```python
from build123d import *

# Parameters (mm, degrees)
BOSS_EXTRUDE1_DEPTH = 40
CUT_EXTRUDE1_REACH  = 4
SKETCH2_R           = 17.5
CUT_EXTRUDE2_REACH  = 4
CUT_EXTRUDE3_REACH  = 4
SKETCH6_R           = 2


with BuildPart() as part:
    # Sketch1 → Boss-Extrude1 (new body)
    with BuildSketch(Plane.XY):
        Polygon((0, 0), (0, 62), (2, 62), (2, 2), (22, 2), (22, 0), align=None)
    extrude(amount=BOSS_EXTRUDE1_DEPTH)

    # Sketch2 → Cut-Extrude1 (cut, up to next)
    with BuildSketch(Plane(origin=(2, 0, 0), x_dir=(0, 0, -1), z_dir=(1, 0, 0)), mode=Mode.PRIVATE) as cut_extrude1_sk1:
        with Locations((-20, 42)):
            Circle(SKETCH2_R)
    cut_extrude1_tool1 = extrude(cut_extrude1_sk1.sketch, amount=-CUT_EXTRUDE1_REACH, mode=Mode.PRIVATE) & part.part
    add(cut_extrude1_tool1.solids().sort_by_distance((2, 42, 20))[0], mode=Mode.SUBTRACT)

    # Sketch5 → Cut-Extrude2 (cut, up to next)
    with BuildSketch(Plane(origin=(2, 0, 0), x_dir=(0, 0, -1), z_dir=(1, 0, 0)), mode=Mode.PRIVATE) as cut_extrude2_sk1:
        with BuildLine():
            Line((-40, 62), (-40, 42))
            ThreePointArc((-40, 42), (-34.142135624, 56.142135624), (-20, 62))
            Line((-20, 62), (-40, 62))
        make_face()
    cut_extrude2_tool1 = extrude(cut_extrude2_sk1.sketch, amount=-CUT_EXTRUDE2_REACH, mode=Mode.PRIVATE) & part.part
    add(cut_extrude2_tool1.solids().sort_by_distance((2, 57.532641, 35.532641))[0], mode=Mode.SUBTRACT)
    # Sketch5 → Cut-Extrude2 (cut, up to next)
    with BuildSketch(Plane(origin=(2, 0, 0), x_dir=(0, 0, -1), z_dir=(1, 0, 0)), mode=Mode.PRIVATE) as cut_extrude2_sk2:
        with BuildLine():
            Line((0, 62), (-20, 62))
            ThreePointArc((-20, 62), (-5.857864376, 56.142135624), (0, 42))
            Line((0, 42), (0, 62))
        make_face()
    cut_extrude2_tool2 = extrude(cut_extrude2_sk2.sketch, amount=-CUT_EXTRUDE2_REACH, mode=Mode.PRIVATE) & part.part
    add(cut_extrude2_tool2.solids().sort_by_distance((2, 57.532641, 4.467359))[0], mode=Mode.SUBTRACT)

    # Sketch6 → Cut-Extrude3 (cut, up to next)
    with BuildSketch(Plane(origin=(0, 2, 0), x_dir=(1, 0, 0), z_dir=(0, 1, 0)), mode=Mode.PRIVATE) as cut_extrude3_sk1:
        with Locations((12, -9)):
            Circle(SKETCH6_R)
    cut_extrude3_tool1 = extrude(cut_extrude3_sk1.sketch, amount=-CUT_EXTRUDE3_REACH, mode=Mode.PRIVATE) & part.part
    add(cut_extrude3_tool1.solids().sort_by_distance((12, 2, 9))[0], mode=Mode.SUBTRACT)
    # Sketch6 → Cut-Extrude3 (cut, up to next)
    with BuildSketch(Plane(origin=(0, 2, 0), x_dir=(1, 0, 0), z_dir=(0, 1, 0)), mode=Mode.PRIVATE) as cut_extrude3_sk2:
        with Locations((12, -31)):
            Circle(SKETCH6_R)
    cut_extrude3_tool2 = extrude(cut_extrude3_sk2.sketch, amount=-CUT_EXTRUDE3_REACH, mode=Mode.PRIVATE) & part.part
    add(cut_extrude3_tool2.solids().sort_by_distance((12, 2, 31))[0], mode=Mode.SUBTRACT)


solid = part.part
```
Read the model definition and answer for the solid it produces. Units are mm, in the model's axes. A direction names the side the tool comes from. Coordinates: 2 decimals unless noted, no trailing zeros. Write each loop counter-clockwise with the first axis right and the second up, starting at its lowest first coordinate (ties: lowest second). Pieces come first, ordered by that corner, then holes. Notation, with made-up numbers: (83.25, 71) - (97.25, 71) arc R17 cw to (97.25, 87) - close; hole circle Ø8 at (38.5, -22). An arc over 180 degrees is marked (long way). Answer as a JSON object with one key per item and string values. Group by question number.
1. A cutting plane is placed at A-A (x = 12). Determine the outline of the cut face in (y, z).
2. The mould has two halves that part along Z. Classify faces 3 (the flat face through (22, 1, 20)), 4 (the cylindrical face through (12, 1, 33)), 5 (the flat face through (1, 15, 0)): +Z half, -Z half, draft (parallel to the pull), parting line (faces both ways), or undercut.
3. Which of the six approach directions +Z, -Z, +X, -X, +Y, -Y give full straight-line access (tool end or side, diameter ignored) to faces 1 (the flat face through (12, 2, 20)), 2 (the cylindrical face through (1.014, 53.827, 32.898))?
4. Consider L1, parallel to Z at x = 12, y = 1.55; L2, parallel to X at y = 1, z = 31; L3, parallel to Y at x = 1.35, z = 20. Determine where each line is inside the solid, lowest interval first. Write a range as [from, to].
5. A cutting plane is placed at D-D (x = 16.25). Determine the outline of the cut face in (y, z).
6. A cutting plane is placed at B-B (z = 5.5). Determine the outline of the cut face in (x, y), plus the area to 3 significant figures.
7. Each of these flat-tipped pins is pushed along its axis until it touches: P1, Ø2, axis at x = 10.5, z = 19.5, coming from the -Y side; P2, Ø3, axis at x = 2.5, z = 33.5, coming from the +Y side; P3, Ø5, axis at x = 10, z = 29.5, coming from the +Y side. Where does it stop, or does it pass through?
8. A cutting plane is placed at C-C (y = 48). Determine the outline of the cut face in (x, z).
Worked out:
{
 "1": {"outline": "(0, 0) - (2, 0) - (2, 7) - (0, 7) - close; (0, 11) - (2, 11) - (2, 29) - (0, 29) - close; (0, 33) - (2, 33) - (2, 40) - (0, 40) - close"},
 "2": {"face 3": "draft", "face 4": "undercut", "face 5": "-Z half"},
 "3": {"face 1": "+Z, -Z, +X, +Y", "face 2": "+X, -X"},
 "4": {"L1": "z = [0, 7], [11, 29], [33, 40]", "L2": "x = [0, 10], [14, 22]", "L3": "y = [0, 24.5], [59.5, 62]"},
 "5": {"outline": "(0, 0) - (2, 0) - (2, 40) - (0, 40) - close"},
 "6": {"outline": "(0, 0) - (22, 0) - (22, 2) - (2, 2) - (2, 32.2) - (0, 32.2) - close; (0, 51.8) - (2, 51.8) - (2, 55.77) - (0, 55.77) - close", "area": "112 mm²"},
 "7": {"P1": "stops at y = 0", "P2": "stops at y = 57.94", "P3": "stops at y = 2"},
 "8": {"outline": "(0, 0.92) - (2, 0.92) - (2, 3.56) - (0, 3.56) - close; (0, 36.44) - (2, 36.44) - (2, 39.08) - (0, 39.08) - close"}
}
